Read the model definition and answer for the solid it produces. Units are mm, in the model's axes. A direction names the side the tool comes from. Give positions to 0.01 mm unless a question says otherwise; leave off trailing zeros. Loops run counter-clockwise (first coordinate to the right, second up) from the corner with the lowest first, then second, coordinate; pieces in that order, holes last. Notation, with made-up numbers: (0, 23.5) - (11, 23.5) arc R20 cw to (11, 34.5) - close; hole circle Ø3 at (-22.5, -8.5). An arc over 180 degrees is marked (long way). Write each question's results on one line, items separated by ' | '. Start each with the question number.
Q1. The part is cut by section B-B, the plane z = 201.5. Write down the section's boundary in (x, y), plus the area to 3 significant figures.
Q2. The part is cut by section A-A, the plane y = 876.3. Write down the section's boundary in (x, z).
Q3. The part is cut by section D-D, the plane z = -138.5. Write down the section's boundary in (x, y), plus the area to 3 significant figures.
Q4. Determine the mould class of faces 1 (the flat face through (584.2, 413, 3)), 2 (the flat face through (-8, 0, -3)), 3 (the cylindrical face through (459.17, 939.77, -203.56)) for opening direction Y: +Y half, -Y half, draft (parallel to the pull), parting line (faces both ways), or undercut.
Q5. Find the intervals of material crossed by line 1 (Y direction, x = 335.5, z = 120.5); line 2 (Y direction, x = -418.5, z = -194), in increasing order. Write a range as from..to.
Q6. The part is cut by section C-C, the plane x = -457.2. Write down the section's boundary in (y, z), plus the area to 3 significant figures.
Q7. For faces 4 (the flat face through (-8, 476, -228.6)), 5 (the flat face through (456, 890, -177.8)), determine the directions among +Z, -Z, +X, -X, +Y, -Y from which every point of the face is accessible in a straight line to the end or side of a thin tool.
Q8. Given pin 1 (5 mm diameter, centred on x = -411.5, z = -154, fed in from +Y), flat-ended and moving along its own axis, determine where the tip first touches the part or whether it passes through.
```python
from build123d import *

# Parameters (mm, degrees)
SKETCH1_W           = 1168.4
SKETCH1_H           = 457.2
BOSS_EXTRUDE1_DEPTH = 838.2
SKETCH2_R           = 63.5
BOSS_EXTRUDE2_DEPTH = 50.8


with BuildPart() as part:
    # Sketch1 → Boss-Extrude1 (new body)
    with BuildSketch(Plane(origin=(0, 0, 0), x_dir=(1, 0, 0), z_dir=(0, 1, 0))):
        Rectangle(SKETCH1_W, SKETCH1_H)
    extrude(amount=BOSS_EXTRUDE1_DEPTH)

    # Sketch2 → Boss-Extrude2 (add)
    with BuildSketch(Plane.XY.offset(228.6)):
        with Locations((-457.2, 876.3)):
            Circle(SKETCH2_R)
        with Locations((457.2, 876.3)):
            Circle(SKETCH2_R)
    boss_extrude2 = extrude(amount=-BOSS_EXTRUDE2_DEPTH)

    # Mirror1: Boss-Extrude2 across plane
    add(boss_extrude2.mirror(Plane.XY))


solid = part.part
```
Check sheet entries:
1) outline: (-584.2, 0) - (584.2, 0) - (584.2, 838.2) - (508, 838.2) arc R63.5 ccw (long way) to (406.4, 838.2) - (-406.4, 838.2) arc R63.5 ccw (long way) to (-508, 838.2) - (-584.2, 838.2) - close | area: 1,000,000 mm^2
2) outline: (-520.7, -228.6) - (-393.7, -228.6) - (-393.7, -177.8) - (-520.7, -177.8) - close; (-520.7, 177.8) - (-393.7, 177.8) - (-393.7, 228.6) - (-520.7, 228.6) - close; (393.7, -228.6) - (520.7, -228.6) - (520.7, -177.8) - (393.7, -177.8) - close; (393.7, 177.8) - (520.7, 177.8) - (520.7, 228.6) - (393.7, 228.6) - close
3) outline: (-584.2, 0) - (584.2, 0) - (584.2, 838.2) - (-584.2, 838.2) - close | area: 979,000 mm^2
4) face 1: draft | face 2: -Y half | face 3: undercut
5) line 1: y = 0..838.2 | line 2: y = 0..926.64
6) outline: (0, -228.6) - (939.8, -228.6) - (939.8, -177.8) - (838.2, -177.8) - (838.2, 177.8) - (939.8, 177.8) - (939.8, 228.6) - (0, 228.6) - close | area: 394,000 mm^2
7) face 4: -Z, +X, -X, +Y, -Y | face 5: +X, -X, +Y
8) pin 1: stops at y = 838.2
